from build123d import *

# Parameters (mm, degrees)
CUT_EXTRUDE3_DEPTH         = 4
DRAFT1_ANGLE               = 20
RECESSI_CUT_EXTRUDE5_DEPTH = 4
SKETCH11_W                 = 5.6
SKETCH11_H                 = 0.666666667
POINT_CUT_EXTRUDE8_DEPTH   = 9


with BuildPart() as part:
    # Sketch1 → base-Revolve (revolve)
    with BuildSketch(Plane.XY):
        with BuildLine():
            Line((0, 0), (0, 4.8))
            ThreePointArc((0, 4.8), (0.9372583, 7.0627417), (3.2, 8))
            Line((3.2, 8), (5.6, 8))
            Line((5.6, 8), (5.6, 3.6))
            ThreePointArc((5.6, 3.6), (5.717157288, 3.317157288), (6, 3.2))
            Line((6, 3.2), (6.8, 3.2))
            Line((6.8, 3.2), (7.6, 4))
            Line((7.6, 4), (25.6, 4))
            Line((25.6, 4), (25.6, 0))
            Line((25.6, 0), (0, 0))
        make_face()
    revolve(axis=Axis((0, 0, 0), (1, 0, 0)))

    # Sketch4 → Cut-Extrude3 (cut)
    with BuildSketch(Plane(origin=(0, 0, 0), x_dir=(0, 0, -1), z_dir=(1, 0, 0))):
        Polygon((0.9, 4.39), (-0.9, 4.39), (-0.9, 0.9), (-4.39, 0.9), (-4.39, -0.9), (-0.9, -0.9), (-0.9, -4.39), (0.9, -4.39), (0.9, -0.9), (4.39, -0.9), (4.39, 0.9), (0.9, 0.9), align=None)
    extrude(amount=CUT_EXTRUDE3_DEPTH, mode=Mode.SUBTRACT)

    # Draft1
    draft1_faces = [part.faces().sort_by_distance(p)[0] for p in [
        (2, 0, -4.39),
        (2, -4.39, 0),
        (2, 0, 4.39),
        (2, 4.39, 0),
    ]]
    draft(draft1_faces, Plane(origin=(0, 0, 0), x_dir=(0, 0, -1), z_dir=(-1, 0, 0)), DRAFT1_ANGLE)

    # Sketch5 → recessI_Cut-Extrude5 (cut)
    with BuildSketch(Plane.ZY):
        Polygon((0.9, 1.778), (1.778, 0.9), (0.9, 0.9), align=None)
        Polygon((-0.9, 0.9), (-1.778, 0.9), (-0.9, 1.778), align=None)
        Polygon((-0.9, -1.778), (-1.778, -0.9), (-0.9, -0.9), align=None)
        Polygon((0.9, -0.9), (1.778, -0.9), (0.9, -1.778), align=None)
    extrude(amount=-RECESSI_CUT_EXTRUDE5_DEPTH, mode=Mode.SUBTRACT)

    # Sketch8 → point_Cut-Revolve1 (revolve, cut)
    with BuildSketch(Plane.XY):
        Polygon((25.6, 0), (26.108, 0), (26.108, 4.508), (24.214359354, 4.508), (24.214359354, 4), (25.6, 3.2), align=None)
    revolve(axis=Axis((0, 0, 0), (1, 0, 0)), mode=Mode.SUBTRACT)

    # Sketch11 → point_Cut-Extrude8 (cut, through all)
    with BuildSketch(Plane.XY):
        with Locations((22.8, -0.333333333)):
            Rectangle(SKETCH11_W, SKETCH11_H)
    extrude(amount=POINT_CUT_EXTRUDE8_DEPTH, mode=Mode.SUBTRACT)


solid = part.part
Design review of the part built by this model. Coordinates are the model's own, in mm. A direction names the side the tool comes from. Coordinates: 2 decimals unless noted, no trailing zeros. Order: outer loops, then holes, each group sorted by start corner. A loop starts at its lowest first (then second) coordinate and runs counter-clockwise, first axis right, second up. Notation, with made-up numbers: (-8, 83) -> (11, 83) arc R22 ccw to (11, 94) -> close; hole circle Ø2 at (30.5, 71.5). An arc over 180 degrees is marked (long way). One line per item, written item: value.
1) Clearance check with flat-ended pins moving along their axes: P1, Ø4.5, axis at x = 23.5, z = 2.5, coming from the -Y side; P2, Ø0.8, axis at x = 1.5, y = 3, coming from the -Z side; P3, Ø8, axis at x = 19, y = 0.5, coming from the -Z side. State where each tip first meets the part, or that it passes through.
Output values:
P1: stops at y = -3.99
P2: stops at z = -7.17
P3: stops at z = -4
2) Draft analysis for pull direction Y (two halves, no side actions). For faces 1 (the face through (23, 0, 2)), 2 (the face through (0, 1.1, -2.1)), 3 (the face through (25.379, 0.136, -3.325)), state which applies: +Y half, -Y half, draft (parallel to the pull), parting line (faces both ways), or undercut.
Output values:
face 1: undercut
face 2: draft
face 3: parting line
3) Machinability: for faces 4 (the face through (23, -0.667, 2)), 5 (the face through (2, -3, -0.9)), which of the approach directions +Z, -Z, +X, -X, +Y, -Y give a long, thin tool a straight path to every point of the face, cutting with its end or side? Answer none if there is none.
Output values:
face 4: +Z, +X
face 5: -X
4) We need section B-B, the plane x = 20.75. Give the boundary of the cut face in (y, z).
Output values:
outline: (-0.67, 0) -> (-0.67, 3.94) arc R4 ccw (long way) to (0, 4) -> (0, 0) -> close
5) We need section A-A, the plane x = 15.25. Give the boundary of the cut face in (y, z), then the cut area to 3 significant figures.
Output values:
outline: circle Ø8 at (0, 0)
area: 50.3 mm2
6) To check wall thickness, follow probe 1 along Z at (x, y) = (17.5, 1.75); probe 2 along X at (y, z) = (-2.5, -3.5); probe 3 along X at (y, z) = (3.75, -1.25). State the ranges of each line that lie inside material, in increasing order. Write a range as [from, to].
Output values:
probe 1: z = [-3.6, 3.6]
probe 2: x = [0, 5.6]
probe 3: x = [0, 5.6], [7.55, 24.3]
